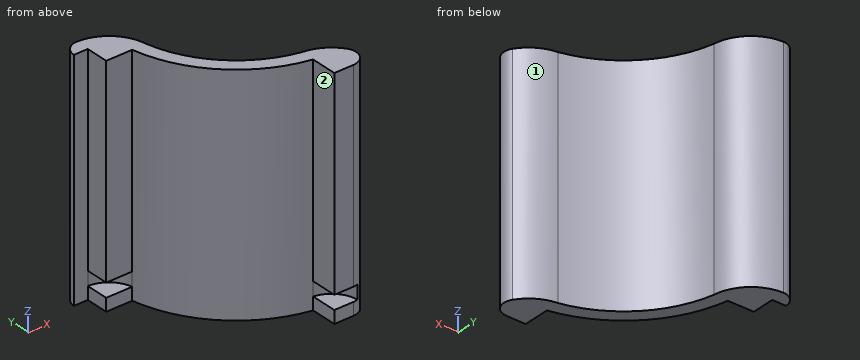
from build123d import *

# Parameters (mm, degrees)
BOSS_EXTRUDE1_DEPTH = 104.775
BOSS_EXTRUDE2_DEPTH = 92.5957
BOSS_EXTRUDE3_START = -5.8293
BOSS_EXTRUDE3_DEPTH = 5.8293
BOSS_EXTRUDE4_DEPTH = 6.35
SKETCH5_W           = 7.787485422
SKETCH5_H           = 19.833751934
SKETCH5_W_2         = 22.754058967
SKETCH5_H_2         = 3.407024872
CUT_EXTRUDE1_DEPTH  = 227.312030137
SKETCH7_W           = 89.459387911
SKETCH7_H           = 93.108081787
CUT_EXTRUDE3_DEPTH  = 104.775
SKETCH8_W           = 104.775
SKETCH8_H           = 6.354337814
BOSS_EXTRUDE5_DEPTH = 6.35
FILLET1_R           = 6.35


with BuildPart() as part:
    # Sketch1 → Boss-Extrude1 (new, symmetric)
    with BuildSketch(Plane.XY):
        with BuildLine():
            Line((-58.2422, 56.2102), (-58.2422, 62.5602))
            ThreePointArc((-58.2422, 62.5602), (-45.640852469, 57.743322347), (-39.3748699, 45.7962))
            ThreePointArc((-39.3748699, 45.7962), (-25.556268964, 20.239931036), (0, 6.4213301))
            ThreePointArc((0, 6.4213301), (12.247457496, 0.293755183), (17.272, -12.446))
            Line((17.272, -12.446), (10.922, -12.446))
            ThreePointArc((10.922, -12.446), (7.760938146, -4.204686933), (0, 0))
            ThreePointArc((0, 0), (-30.011530905, 15.784669095), (-45.7962, 45.7962))
            ThreePointArc((-45.7962, 45.7962), (-50.144819563, 53.243313205), (-58.2422, 56.2102))
        make_face()
    extrude(amount=BOSS_EXTRUDE1_DEPTH, both=True)


with BuildPart() as boss_extrude2_tool:
    # Sketch2 → Boss-Extrude2 (new, symmetric)
    with BuildSketch(Plane.XY):
        with BuildLine():
            Line((-58.2422, 56.2102), (-58.2422, 45.796198296))
            Line((-58.2422, 45.796198296), (-45.796199685, 45.796198296))
            ThreePointArc((-45.796199685, 45.796198296), (-50.144818899, 53.243312648), (-58.2422, 56.2102))
        make_face()
        with BuildLine():
            Line((0, 0), (0, -12.446))
            Line((0, -12.446), (10.922, -12.446))
            ThreePointArc((10.922, -12.446), (7.760938146, -4.204686933), (0, 0))
        make_face()
    extrude(amount=BOSS_EXTRUDE2_DEPTH, both=True)


with BuildPart() as part_1:
    add(part.part)


with BuildPart() as part_2:
    # Boss-Extrude2: joined with boss_extrude2_tool
    add(part_1.part.fuse(boss_extrude2_tool.part, tol=0.00001))

    # Sketch3 → Boss-Extrude3 (add)
    with BuildSketch(Plane(origin=(0, 0, -104.775), x_dir=(-1, 0, 0), z_dir=(0, 0, -1)).offset(BOSS_EXTRUDE3_START)):
        with BuildLine():
            Line((58.2422, 56.2102), (58.2422, 45.796198296))
            Line((58.2422, 45.796198296), (45.7962, 45.7962))
            ThreePointArc((45.7962, 45.7962), (50.144819563, 53.243313205), (58.2422, 56.2102))
        make_face()
        with BuildLine():
            Line((0, 0), (0, -12.446))
            Line((0, -12.446), (-10.922, -12.446))
            ThreePointArc((-10.922, -12.446), (-7.760938146, -4.204686933), (0, 0))
        make_face()
    extrude(amount=BOSS_EXTRUDE3_DEPTH)

    # Sketch4 → Boss-Extrude4 (add)
    with BuildSketch(Plane.XY.offset(104.775)):
        with BuildLine():
            Line((-58.2422, 56.2102), (-58.2422, 45.796198296))
            Line((-58.2422, 45.796198296), (-45.7962, 45.7962))
            ThreePointArc((-45.7962, 45.7962), (-50.144819563, 53.243313205), (-58.2422, 56.2102))
        make_face()
        with BuildLine():
            Line((0, 0), (0, -12.446))
            Line((0, -12.446), (10.922, -12.446))
            ThreePointArc((10.922, -12.446), (7.760938146, -4.204686933), (0, 0))
        make_face()
    extrude(amount=-BOSS_EXTRUDE4_DEPTH)

    # Sketch5 → Cut-Extrude1 (cut, through all)
    with BuildSketch(Plane.XY.offset(104.775)):
        with Locations((-61.627942711, 54.680509116)):
            Rectangle(SKETCH5_W, SKETCH5_H)
        with Locations((8.225058429, -13.641512436)):
            Rectangle(SKETCH5_W_2, SKETCH5_H_2)
    extrude(amount=-CUT_EXTRUDE1_DEPTH, mode=Mode.SUBTRACT)

    # Sketch7 → Cut-Extrude3 (cut)
    with BuildSketch(Plane.XY.offset(104.775)):
        with Locations((-22.903611999, 28.130063449)):
            Rectangle(SKETCH7_W, SKETCH7_H)
    extrude(amount=-CUT_EXTRUDE3_DEPTH, mode=Mode.SUBTRACT)

    # Sketch8 → Boss-Extrude5 (add)
    with BuildSketch(Plane.ZY.offset(57.7342)):
        with Locations((-52.3875, 59.374341949)):
            Rectangle(SKETCH8_W, SKETCH8_H)
    extrude(amount=BOSS_EXTRUDE5_DEPTH)

    # Fillet1
    # the kernel refuses this fillet: 6.35 mm, written as the material it takes off along each edge
    with BuildSketch(Plane(origin=(17.260151367, -11.938, -130.624178653), x_dir=(-0.30497213299383213, 0.9523612749882223, 0), z_dir=(0, 0, 1))) as fillet1_piece_1:
        with BuildLine():
            CenterArc((8.625598356, 6.114282737), FILLET1_R, 162.243512631, 123.416753829)
            Line((2.57810426, 8.050855782), (0, 0))
            ThreePointArc((0, 0), (5.169835731, -0.710949564), (10.339671461, 0))
        make_face()
    extrude(amount=156.473357306, mode=Mode.SUBTRACT)
    with BuildSketch(Plane(origin=(-64.0842, 62.551510856, -120.65), x_dir=(1, 0, 0), z_dir=(0, 0, 1))) as fillet1_piece_2:
        with BuildLine():
            CenterArc((FILLET1_R, -FILLET1_R), FILLET1_R, 90, 90)
            Line((0, -FILLET1_R), (0, 0))
            Line((0, 0), (FILLET1_R, 0))
        make_face()
    extrude(amount=136.525, mode=Mode.SUBTRACT)


solid = part_2.part
Work out the finished part from the listing and answer in its coordinate system (mm). Face numbers are marked on the shaded views. A direction names the side the tool comes from. Coordinates: 2 decimals unless noted, no trailing zeros. Write each loop counter-clockwise with the first axis right and the second up, starting at its lowest first coordinate (ties: lowest second). Pieces come first, ordered by that corner, then holes. Notation, with made-up numbers: M -38.75,86.5 L 19.25,86.5 A8 ccw 19.25,93.5 Z; hole C -11.75,14.5 d6. An arc over 180 degrees is marked long. Use one line per item in the form item = value. Start each with the question number.
1. Straight lines are drawn through the part: probe 1 along Z at (x, y) = (-50, 47.5) (3 decimals); probe 2 along X at (y, z) = (-5.5, -55.5); probe 3 along Y at (x, z) = (-2, -40.5). For each, find the intervals that lie inside material, in ascending order. Write a range as from..to.
2. A tool of negligible diameter and unlimited length cuts with its end or side. For the marked faces 1 and 2, from which of +Z, -Z, +X, -X, +Y, -Y can it reach the whole face along a straight path? Write none if from no direction.
3. The part is cut by section C-C (y = 14.5). Give the vertices of the cut face in (x, z) (3 decimals), plus the area to 3 significant figures.
4. The part is cut by section B-B (x = 6). Give the vertices of the cut face in (y, z) (3 decimals).
5. The part is cut by section D-D (x = -48.5). Give the vertices of the cut face in (y, z) (3 decimals).
6. Each of these flat-tipped pins is pushed along its axis until it touches: P1, Ø3, axis at y = 49, z = -102, coming from the -X side; P2, Ø10, axis at x = -38.5, z = -25.5, coming from the +Y side; P3, Ø1.9, axis at x = -60, z = -59.5, coming from the -Y side. Where does it stop, or does it pass through?
Evaluation:
q1.probe_1 = -104.775..-98.946, -92.596..0
q1.probe_2 = 0..15.16
q1.probe_3 = 0.41..6.88
q2.face_1 = +Z, -Z, +X, +Y
q2.face_2 = +Z, -Z, -X, -Y
q3.outline = M -28.685,-104.775 L -18.706,-104.775 L -18.706,0 L -28.685,0 Z
q3.area = 1,050 mm^2
q4.outline = M -11.938,-104.775 L 4.818,-104.775 L 4.818,0 L -11.938,0 L -11.938,-92.596 L -2.546,-92.596 L -2.546,-98.946 L -11.938,-98.946 Z
q5.outline = M 45.796,-104.775 L 59.843,-104.775 L 59.843,0 L 45.796,0 L 45.796,-92.596 L 51.588,-92.596 L 51.588,-98.946 L 45.796,-98.946 Z
q6.P1 = -57.73
q6.P2 = 55.5
q6.P3 = 56.2
